Part model, mm, in its own coordinate system. Coordinates: 2 decimals unless noted, no trailing zeros. Loops run counter-clockwise (first coordinate to the right, second up) from the corner with the lowest first, then second, coordinate; pieces in that order, holes last. Notation, with made-up numbers: M 74,7 L 125,7 A12 cw 125,16 Z; hole C 15,50.25 d6. An arc over 180 degrees is marked long. Answer as a JSON object with one key per item and string values. Group by question number.
1. Saw through at A-A on x = 0. Write the cut outline in (y, z).
2. Drop a flat-ended pin along its axis: pin 1 Ø5 at (x, z) = (-35.5, 35.5) entering from -Y. Give the stop position or say it passes through.
3. Saw through at D-D on z = 35.5. Write the cut outline in (x, y), then the cut area to 3 significant figures.
4. Drill centre lines: L1, parallel to Z at x = -18.5, y = 1.35; L2, parallel to X at y = 0.2, z = 0.5; L3, parallel to X at y = 1.4, z = -35.5. Where is each one in solid material? Low to high.
5. Mould opens along X. For faces 1 (the face through (-40.135, 0.902, -40.603)), 2 (the face through (-26, 1.83, 37)), 3 (the face through (-34.75, 0.9, 33.7)), 4 (the face through (25.404, 0.902, 33.131)) say: released by +X, released by -X, zero draft, split by the parting line, or undercut.
6. Saw through at C-C on y = 0.55. Write the cut outline in (x, z).
7. Saw through at B-B on z = 0. Write the cut outline in (x, y), then the cut area to 3 significant figures.
from build123d import *

# Parameters (mm, degrees)
BOSS_EXTRUDE1_DEPTH = 1.83
SKETCH2_R           = 1.95
SKETCH2_R_2         = 41.75
CUT_EXTRUDE1_DEPTH  = 23.83


with BuildPart() as part:
    # Sketch1 → Boss-Extrude1 (new body)
    with BuildSketch(Plane(origin=(0, 0, 0), x_dir=(1, 0, 0), z_dir=(0, 1, 0))):
        Polygon((57.09, -23.647452276), (57.09, 23.647452276), (23.647452276, 57.09), (-23.647452276, 57.09), (-57.09, 23.647452276), (-57.09, -23.647452276), (-23.647452276, -57.09), (23.647452276, -57.09), align=None)
    extrude(amount=BOSS_EXTRUDE1_DEPTH)

    # Sketch2 → Cut-Extrude1 (cut)
    with BuildSketch(Plane(origin=(0, 0, 0), x_dir=(1, 0, 0), z_dir=(0, 1, 0))):
        with Locations(Location((-35.5, 35.5, 0), (0, 0, 90))):
            Circle(SKETCH2_R)
        with Locations(Location((35.5, 35.5, 0), (0, 0, 90))):
            Circle(SKETCH2_R)
        with Locations(Location((35.5, -35.5, 0), (0, 0, 90))):
            Circle(SKETCH2_R)
        with Locations(Location((-35.5, -35.5, 0), (0, 0, 90))):
            Circle(SKETCH2_R)
        with Locations(Location((0, 0, 0), (0, 0, 90))):
            Circle(SKETCH2_R_2)
    extrude(amount=CUT_EXTRUDE1_DEPTH, mode=Mode.SUBTRACT)


solid = part.part
Outcome:
{
 "1": {"outline": "M 0,-57.09 L 1.83,-57.09 L 1.83,-41.75 L 0,-41.75 Z; M 0,41.75 L 1.83,41.75 L 1.83,57.09 L 0,57.09 Z"},
 "2": {"pin 1": "stops at y = 0"},
 "3": {"outline": "M -45.24,0 L -37.45,0 L -37.45,1.83 L -45.24,1.83 Z; M -33.55,0 L -21.97,0 L -21.97,1.83 L -33.55,1.83 Z; M 21.97,0 L 33.55,0 L 33.55,1.83 L 21.97,1.83 Z; M 37.45,0 L 45.24,0 L 45.24,1.83 L 37.45,1.83 Z", "area": "70.9 mm²"},
 "4": {"L1": "z = -57.09 to -37.43, 37.43 to 57.09", "L2": "x = -57.09 to -41.75, 41.75 to 57.09", "L3": "x = -45.24 to -37.45, -33.55 to -21.97, 21.97 to 33.55, 37.45 to 45.24"},
 "5": {"face 1": "released by -X", "face 2": "zero draft", "face 3": "undercut", "face 4": "undercut"},
 "6": {"outline": "M -57.09,-23.65 L -23.65,-57.09 L 23.65,-57.09 L 57.09,-23.65 L 57.09,23.65 L 23.65,57.09 L -23.65,57.09 L -57.09,23.65 Z; hole C 0,0 d83.5; hole C -35.5,-35.5 d3.9; hole C -35.5,35.5 d3.9; hole C 35.5,-35.5 d3.9; hole C 35.5,35.5 d3.9"},
 "7": {"outline": "M -57.09,0 L -41.75,0 L -41.75,1.83 L -57.09,1.83 Z; M 41.75,0 L 57.09,0 L 57.09,1.83 L 41.75,1.83 Z", "area": "56.1 mm²"}
}
